Autodesk Inventor part; units mm, degrees
sketch "Sketch1" plane through (0, 0, 0) normal (0, 0, 1) x (1, 0, 0)
  circle A0 centre (-76.2, 0) radius 15.875
  line L0 (-38.1, 0) -> (38.1, 0) construction
  line L1 (-38.1, -6.35) -> (38.1, -6.35)
  line L2 (38.1, 6.35) -> (-38.1, 6.35)
  arc A1 (-38.1, 6.35) -> (-38.1, -6.35) centre (-38.1, 0) ccw
  arc A2 (38.1, -6.35) -> (38.1, 6.35) centre (38.1, 0) ccw
  arc A3 (88.9, 31.75) -> (88.9, -31.75) centre (88.9, 0) ccw
  circle A4 centre (-76.2, 0) radius 12.7
  arc A5 (88.9, 25.4) -> (88.9, -25.4) centre (88.9, 0) ccw
  line L3 (88.9, 31.75) -> (88.9, 25.4)
  line L4 (88.9, -25.4) -> (88.9, -31.75)
  line L5 (88.9, 31.75) -> (69.85, 31.75)
  line L6 (88.9, -31.75) -> (69.85, -31.75)
  line L7 (-58.2395, 9.525) -> (27.8487, 9.525)
  line L8 (-58.2395, -9.525) -> (27.8487, -9.525)
  arc A6 (27.8487, 9.525) -> (69.85, 31.75) centre (27.8487, 60.325) ccw
  arc A7 (69.85, -31.75) -> (27.8487, -9.525) centre (27.8487, -60.325) ccw
  arc A8 (-66.2219, 12.3472) -> (-58.2395, 9.525) centre (-58.2395, 22.225) ccw
  arc A9 (-58.2395, -9.525) -> (-66.2219, -12.3472) centre (-58.2395, -22.225) ccw
  point P0 (0, 0)
  point P1 (0, 0)
  dimension "d0" = 31.75
  dimension "d1" = 25.4
  dimension "d2" = 12.7
  dimension "d3" = 76.2
  dimension "d4" = 165.1
  dimension "d5" = 50.8
  dimension "d6" = 63.5
  dimension "d7" = 50.8
  dimension "d8" = 19.05
  dimension "d9" = 19.05
  dimension "d12" = 19.05
  dimension "d13" = 9.525
  dimension "d15" = 101.6
  dimension "d16" = 101.6
  dimension "d18" = 25.4
  dimension "d19" = 0
  dimension "d39" = 31.75
  dimension "d41" = 25.4
extrude "Base" add sketch "Sketch1" along normal mid plane 12.7
extrude "Indent" add sketch "Sketch1" along normal mid plane 6.35 contours A1 L2 A2 L1
extrude "Extrusion4" add sketch "Sketch1" along normal mid plane 25.4 contours L3 A5 L4 A3
sketch "Sketch3" plane through (88.9, 25.4, 12.7) normal (1, 0, 0) x (0, 0, -1)
  line L0 (6.35, 6.35) -> (19.05, 6.35)
  line L1 (19.05, 6.35) -> (19.05, 12.7)
  line L2 (6.35, 12.7) -> (6.35, 6.35)
  line L3 (6.35, 6.35) -> (19.05, 6.35)
  line L4 (0, 0) -> (0, 6.35)
  line L5 (25.4, 0) -> (0, 0)
  line L6 (25.4, 6.35) -> (25.4, 0)
  arc A0 (19.05, 12.7) -> (6.35, 12.7) centre (12.7, 12.7) ccw
  circle A1 centre (12.7, 12.7) radius 3.175
  line L7 (-5.08, -25.4) -> (30.48, -25.4)
  line L8 (6.35, -57.15) -> (19.05, -57.15)
  line L9 (19.05, -57.15) -> (19.05, -63.5)
  line L10 (6.35, -63.5) -> (6.35, -57.15)
  line L11 (6.35, -57.15) -> (19.05, -57.15)
  line L12 (6.35, -57.15) -> (19.05, -57.15)
  arc A2 (6.35, -63.5) -> (19.05, -63.5) centre (12.7, -63.5) ccw
  circle A3 centre (12.7, -63.5) radius 3.175
  line L13 (6.35, 6.35) -> (19.05, 6.35)
  line L14 (19.05, 6.35) -> (25.4, 6.35)
  line L15 (0, 6.35) -> (6.35, 6.35)
  point P0 (12.7, -25.4)
  dimension "d28" = 0
  dimension "d30" = 12.7
  dimension "d31" = 6.35
  dimension "d32" = 6.35
  dimension "d42" = 6.35
  dimension "d43" = 76.2
  dimension "d44" = 6.35
extrude "Extrusion5" add sketch "Sketch3" against normal blind 12.7 contours L2 A0 L1 L0 | L8 L9 A2 L10
sketch "Sketch4" plane through (0, 0, 6.35) normal (0, 0, 1) x (1, 0, 0)
  arc A0 (-66.2219, 12.3472) -> (-66.2219, -12.3472) centre (-76.2, 0) ccw
  circle A1 centre (-76.2, 0) radius 12.7
  circle A2 centre (-76.2, 0) radius 12.7
  circle A3 centre (-76.2, 0) radius 15.875
  arc A4 (88.9, 31.75) -> (88.9, -31.75) centre (88.9, 0) ccw
  line L0 (88.9, 38.1) -> (88.9, 31.75)
  line L1 (88.9, 38.1) -> (76.2, 38.1)
  line L2 (76.2, 31.75) -> (76.2, 38.1)
  line L3 (76.2, 31.75) -> (69.85, 31.75)
  arc A5 (27.8487, 9.525) -> (69.85, 31.75) centre (27.8487, 60.325) ccw
  line L4 (27.8487, 9.525) -> (-58.2395, 9.525)
  arc A6 (-66.2219, 12.3472) -> (-58.2395, 9.525) centre (-58.2395, 22.225) ccw
  arc A7 (-58.2395, -9.525) -> (-66.2219, -12.3472) centre (-58.2395, -22.225) ccw
  line L5 (-58.2395, -9.525) -> (27.8487, -9.525)
  arc A8 (69.85, -31.75) -> (27.8487, -9.525) centre (27.8487, -60.325) ccw
  line L6 (69.85, -31.75) -> (76.2, -31.75)
  line L7 (76.2, -38.1) -> (76.2, -31.75)
  line L8 (88.9, -38.1) -> (76.2, -38.1)
  line L9 (88.9, -31.75) -> (88.9, -38.1)
  point P0 (0, 0)
extrude "Extrusion6" add sketch "Sketch4" against normal blind 19.05 and the other way blind 6.35 contours A3 A0
properties part number "7.3_Connecting_Rod"
For this review, take the finished solid that the model builds, in its own axes (mm). A direction names the side the tool comes from. Round coordinates to 2 decimals unless told otherwise and drop trailing zeros. Order: outer loops, then holes, each group sorted by start corner. A loop starts at its lowest first (then second) coordinate and runs counter-clockwise, first axis right, second up.
Q1. We need section B-B, the plane z = 9.75. Give the boundary of the cut face in (x, y) (3 decimals), plus the area to 3 significant figures.
Findings below:
outline: circle Ø31.75 at (-76.2, 0); (88.9, -31.75) - (88.9, -25.4) arc R25.4 cw to (88.9, 25.4) - (88.9, 31.75) arc R31.75 ccw to start; hole circle Ø25.4 at (-76.2, 0)
area: 855 mm2
Q2. Wall thickness on line 1 (Y direction, x = -76.2, z = -6.25) (3 decimals); line 2 (Y direction, x = 16, z = 5.25) (3 decimals); line 3 (Y direction, x = 86, z = 0) (3 decimals): over which ranges is each line inside the solid? List them lowest first.
Findings below:
line 1: y = -15.875 to -12.7, 12.7 to 15.875
line 2: y = -9.525 to -6.35, 6.35 to 9.525
line 3: y = -44.45 to -41.275, -34.925 to -25.234, 25.234 to 34.925, 41.275 to 44.45
Q3. Insertion check: P1, Ø1, axis at x = -5, z = 5, coming from the +Y side (3 decimals); P2, Ø14, axis at x = -15, z = -1.5, coming from the -Y side (3 decimals); P3, Ø6.5, axis at y = -38.5, z = 2, coming from the -X side. Each pin has a flat end and moves straight along its axis. Give the tip position at first contact, or say it passes through.
Findings below:
P1: stops at y = 9.525
P2: stops at y = -9.525
P3: stops at x = 76.2
Q4. We need section D-D, the plane x = 0.5. Give the boundary of the cut face in (y, z) (3 decimals).
Findings below:
outline: (-9.525, -6.35) - (-6.35, -6.35) - (-6.35, -3.175) - (6.35, -3.175) - (6.35, -6.35) - (9.525, -6.35) - (9.525, 6.35) - (6.35, 6.35) - (6.35, 3.175) - (-6.35, 3.175) - (-6.35, 6.35) - (-9.525, 6.35) - close
Q5. We need section A-A, the plane z = 0. State how many separate pieces and enclosed holes the cut face has, plus the area to 3 significant figures.
Findings below:
separate pieces: 3
enclosed holes: 1
area: 3,700 mm2
Q6. We need section C-C, the plane y = 4. Give the boundary of the cut face in (x, z) (3 decimals).
Findings below:
outline: (-91.563, -12.7) - (-88.254, -12.7) - (-88.254, 12.7) - (-91.563, 12.7) - (-91.563, -6.35) - close; (-64.146, -12.7) - (-60.837, -12.7) - (-60.837, -6.35) - (-43.032, -6.35) - (-43.032, -3.175) - (43.032, -3.175) - (43.032, -6.35) - (57.403, -6.35) - (57.403, -12.7) - (63.817, -12.7) - (63.817, 12.7) - (57.403, 12.7) - (57.403, 6.35) - (43.032, 6.35) - (43.032, 3.175) - (-43.032, 3.175) - (-43.032, 6.35) - (-60.837, 6.35) - (-60.837, 12.7) - (-64.146, 12.7) - close
Q7. Machinability: for faces 1 (the flat face through (73, -31.75, 0)), 2 (the cylindrical face through (44.45, 0.14, 4.74)), 3 (the cylindrical face through (-44.45, -0.14, -4.78)), which of the approach directions +Z, -Z, +X, -X, +Y, -Y give a long, thin tool a straight path to every point of the face, cutting with its end or side? Answer none if there is none.
Findings below:
face 1: +Z, -Z, -X, -Y
face 2: +Z
face 3: -Z
Q8. Mouldability with a two-part tool opening along Z and no side actions: class faces 4 (the cylindrical face through (82.64, 35, 0.69)), 5 (the cylindrical face through (82.64, -44.45, 0.14)), 6 (the cylindrical face through (-62.416, 10.231, -0.089)) as pulls with the +Z half, pulls with the -Z half, needs draft (parallel to the pull), parting line crosses it, or undercut.
Findings below:
face 4: undercut
face 5: parting line crosses it
face 6: needs draft
